Model file for the job. Use its own axes, mm. A direction names the side the tool comes from. Round coordinates to 2 decimals unless told otherwise and drop trailing zeros. Order: outer loops, then holes, each group sorted by start corner. A loop starts at its lowest first (then second) coordinate and runs counter-clockwise, first axis right, second up. Notation, with made-up numbers: M 81,58 L 107,58 A24 ccw 107,85 Z; hole C 76,23.5 d4. An arc over 180 degrees is marked long. Return JSON: item names as keys, results as strings. Group by question number.
Item 1: Slice it at A-A on y = -2.5. Write the cut outline in (x, z).
Item 2: Probe line 1 along X through (y, z) = (0, 11); line 2 along X through (y, z) = (0, 8); line 3 along Y through (x, z) = (9.5, 16.65). List the from-to ranges inside material, lowest first.
Item 3: Slice it at B-B on z = 4.75. Give the number of separate pieces and of enclosed holes in the cut face, then the cut area to 3 significant figures.
Item 4: Which spindle directions (+Z, -Z, +X, -X, +Y, -Y) get a long thin tool onto all of the face, cutting with end or side? Do faces 5 (the face through (-8, -1, 14)), 6 (the face through (6, -13, 9)), 7 (the face through (-8, -3.5, 9)). Say none if no direction does.
Item 5: Slice it at D-D on y = -16. Write the cut outline in (x, z).
Item 6: Slice it at C-C on x = -1.25. Write the cut outline in (y, z).
Item 7: Pin check, flat tips, straight feed: pin 1 Ø1 at (x, z) = (-9.5, 3) entering from +Y; pin 2 Ø2.5 at (y, z) = (2.5, 11.5) entering from +X; pin 3 Ø1.5 at (x, y) = (7.5, 14) entering from +Z; pin 4 Ø9 at (y, z) = (15, 5) entering from -X. Stop position of each tip, or through.
Item 8: Pull direction X, two halves, no side cores. Call faces 1 (the face through (0, 2.5, 17)), 2 (the face through (0, 0, 0)), 3 (the face through (4, 1, 13)), 4 (the face through (6, 12, 9)): pulls with the +X half, pulls with the -X half, needs draft (parallel to the pull), parting line crosses it, or undercut.
from build123d import *

# Parameters (mm, degrees)
SKETCH1_R                       = 3.5
SKETCH1_R_2                     = 1.65
BOSS_EXTRUDE1_DEPTH             = 17.5
FILLET1_R                       = 0.25
SKIZZE1_W                       = 8
SKIZZE1_H                       = 5
SCHNITT_LINEAR_AUSTRAGEN1_DEPTH = 8
SKIZZE2_W                       = 8
SKIZZE2_H                       = 4
SCHNITT_LINEAR_AUSTRAGEN2_DEPTH = 10
VERRUNDUNG1_R                   = 3
SKIZZE3_R                       = 3
SCHNITT_LINEAR_AUSTRAGEN3_DEPTH = 3.5


with BuildPart() as part:
    # Sketch1 → Boss-Extrude1 (new body)
    # profile 1 of 7: a face of its own
    with BuildSketch(Plane.XY):
        with BuildLine():
            Line((-6, -3.5), (-6, -23.75))
            ThreePointArc((-6, -23.75), (0, -17.75), (6, -23.75))
            Line((6, -23.75), (6, -3.5))
            Line((6, -3.5), (6, 1e-09))
            Line((6, 1e-09), (6, 3.5))
            Line((6, 3.5), (6, 23.75))
            ThreePointArc((6, 23.75), (0, 17.75), (-6, 23.75))
            Line((-6, 23.75), (-6, 3.5))
            Line((-6, 3.5), (-6, 0))
            Line((-6, 0), (-6, -3.5))
        make_face()
    # profile 2 of 7: a face of its own
    with BuildSketch(Plane.XY):
        with BuildLine():
            ThreePointArc((-9.5, 3.5), (-7.025126266, 2.474873734), (-6, 0))
            Line((-6, 0), (-6, 3.5))
            Line((-6, 3.5), (-9.5, 3.5))
        make_face()
    # profile 3 of 7: a face of its own
    with BuildSketch(Plane.XY):
        with BuildLine():
            Line((-9.5, -3.5), (-6, -3.5))
            Line((-6, -3.5), (-6, 0))
            ThreePointArc((-6, 0), (-7.025126266, -2.474873734), (-9.5, -3.5))
        make_face()
    # profile 4 of 7: a face of its own
    with BuildSketch(Plane.XY):
        with Locations((-9.5, 0)):
            Circle(SKETCH1_R)
        with Locations((-9.5, 0)):
            Circle(SKETCH1_R_2, mode=Mode.SUBTRACT)
    # profile 5 of 7: a face of its own
    with BuildSketch(Plane.XY):
        with Locations((9.5, 0)):
            Circle(SKETCH1_R)
        with Locations((9.5, 0)):
            Circle(SKETCH1_R_2, mode=Mode.SUBTRACT)
    # profile 6 of 7: a face of its own
    with BuildSketch(Plane.XY):
        with BuildLine():
            Line((6, 3.5), (6, 1e-09))
            ThreePointArc((6, 1e-09), (7.025126266, 2.474873734), (9.5, 3.5))
            Line((9.5, 3.5), (6, 3.5))
        make_face()
    # profile 7 of 7: a face of its own
    with BuildSketch(Plane.XY):
        with BuildLine():
            Line((6, 1e-09), (6, -3.5))
            Line((6, -3.5), (9.5, -3.5))
            ThreePointArc((9.5, -3.5), (7.025126266, -2.474873734), (6, 1e-09))
        make_face()
    extrude(amount=BOSS_EXTRUDE1_DEPTH)

    # Fillet1
    fillet1_edges = [part.edges().sort_by_distance(p)[0] for p in [
        (-6, 23.75, 8.75),
        (6, 23.75, 8.75),
        (6, -23.75, 8.75),
    ]]
    fillet(fillet1_edges, radius=FILLET1_R)
    fillet1_2_edges = [part.edges().sort_by_distance(p)[0] for p in [
        (-6, -23.75, 8.75),
    ]]
    fillet(fillet1_2_edges, radius=FILLET1_R)

    # Skizze1 → Schnitt-Linear austragen1 (cut)
    with BuildSketch(Plane.XY.offset(17.5)):
        with Locations((0, 5)):
            Rectangle(SKIZZE1_W, SKIZZE1_H)
    extrude(amount=-SCHNITT_LINEAR_AUSTRAGEN1_DEPTH, mode=Mode.SUBTRACT)

    # Skizze2 → Schnitt-Linear austragen2 (cut)
    with BuildSketch(Plane(origin=(0, 2.5, 0), x_dir=(1, 0, 0), z_dir=(0, 1, 0))):
        with Locations((0, -11.5)):
            Rectangle(SKIZZE2_W, SKIZZE2_H)
    extrude(amount=-SCHNITT_LINEAR_AUSTRAGEN2_DEPTH, mode=Mode.SUBTRACT)

    # Verrundung1
    verrundung1_edges = [part.edges().sort_by_distance(p)[0] for p in [
        (0, 2.5, 13.5),
        (0, 7.5, 17.5),
    ]]
    fillet(verrundung1_edges, radius=VERRUNDUNG1_R)

    # Skizze3 → Schnitt-Linear austragen3 (cut)
    with BuildSketch(Plane.XY.offset(17.5)):
        with Locations((-9.5, 0)):
            Circle(SKIZZE3_R)
        with Locations((9.5, 0)):
            Circle(SKIZZE3_R)
    extrude(amount=-SCHNITT_LINEAR_AUSTRAGEN3_DEPTH, mode=Mode.SUBTRACT)


solid = part.part
Output values:
{
 "1": {"outline": "M -11.95,0 L 11.95,0 L 11.95,17.5 L 11.16,17.5 L 11.16,14 L 7.84,14 L 7.84,17.5 L -7.84,17.5 L -7.84,14 L -11.16,14 L -11.16,17.5 L -11.95,17.5 Z; hole M -4,9.5 L 4,9.5 L 4,13.5 L -4,13.5 Z"},
 "2": {"line 1": "-13 to -11.15, -7.85 to -4, 4 to 7.85, 11.15 to 13", "line 2": "-13 to -11.15, -7.85 to 7.85, 11.15 to 13", "line 3": "-3.5 to -3, 3 to 3.5"},
 "3": {"separate pieces": "1", "enclosed holes": "2", "area": "526 mm²"},
 "4": {"face 5": "+Z", "face 6": "+Z, -Z, +X, -Y", "face 7": "+Z, -Z, -X, -Y"},
 "5": {"outline": "M -6,0 L 6,0 L 6,17.5 L -6,17.5 Z"},
 "6": {"outline": "M -17.88,0 L 17.88,0 L 17.88,17.5 L 10.5,17.5 A3 ccw 7.5,14.5 L 7.5,9.5 L -7.5,9.5 L -7.5,13.5 L -0.5,13.5 A3 ccw 2.5,16.5 L 2.5,17.5 L -17.88,17.5 Z"},
 "7": {"pin 1": "y = 3.5", "pin 2": "x = 12.77", "pin 3": "through", "pin 4": "x = -6"},
 "8": {"face 1": "undercut", "face 2": "needs draft", "face 3": "undercut", "face 4": "pulls with the +X half"}
}
